from build123d import *

# Parameters (mm, degrees)
EXTRUDE_1_DEPTH     = 100
SKETCH_2_R          = 11.5
EXTRUDE_2_DEPTH     = 10
SKETCH_3_W          = 23
SKETCH_3_H          = 11.5
EXTRUDE_3_DEPTH     = 20
FILLET_3_R          = 4
FILLET_4_R          = 4
CUT_EXTRUDE_1_DEPTH = 132.291660154
EXTRUDE_4_DEPTH     = 11.5
CUT_EXTRUDE_2_DEPTH = 20
CUT_EXTRUDE_3_DEPTH = 5
SKETCH_8_R          = 1.5
CUT_EXTRUDE_4_DEPTH = 133.303102986


with BuildPart() as part:
    # 草图1 → 凸台-拉伸1 (new body)
    with BuildSketch(Plane.XY):
        with BuildLine():
            Line((-7.5, 12.990381057), (7.5, 12.990381057))
            ThreePointArc((7.5, 12.990381057), (10.606601718, 10.606601718), (12.990381057, 7.5))
            Line((12.990381057, 7.5), (12.990381057, -7.5))
            ThreePointArc((12.990381057, -7.5), (10.606601718, -10.606601718), (7.5, -12.990381057))
            Line((7.5, -12.990381057), (-7.5, -12.990381057))
            ThreePointArc((-7.5, -12.990381057), (-10.606601718, -10.606601718), (-12.990381057, -7.5))
            Line((-12.990381057, -7.5), (-12.990381057, 7.5))
            ThreePointArc((-12.990381057, 7.5), (-10.606601718, 10.606601718), (-7.5, 12.990381057))
        make_face()
    extrude(amount=EXTRUDE_1_DEPTH)

    # 草图2 → 凸台-拉伸2 (add)
    with BuildSketch(Plane.XY.offset(100)):
        Circle(SKETCH_2_R)
    extrude(amount=EXTRUDE_2_DEPTH)

    # 草图3 → 凸台-拉伸3 (add)
    with BuildSketch(Plane.XY.offset(110)):
        with Locations((0, -5.75)):
            Rectangle(SKETCH_3_W, SKETCH_3_H)
    extrude(amount=EXTRUDE_3_DEPTH)

    # 圆角3
    # the kernel refuses this fillet: 4 mm, written as the material it adds along each edge
    with BuildSketch(Plane(origin=(0, 0, 110), x_dir=(0, -1, 0), z_dir=(-1, 0, 0))) as fillet_3_piece_1_section:
        with BuildLine():
            CenterArc((11.5 + FILLET_3_R, -FILLET_3_R), FILLET_3_R, 90, 90)
            Line((11.5 + FILLET_3_R, 0), (11.5, 0))
            Line((11.5, 0), (11.5, -FILLET_3_R))
        make_face()
    fillet_3_piece_1 = revolve(axis=Axis((0, 0, 110), (0, 0, 1)), revolution_arc=90, mode=Mode.PRIVATE)
    fillet_3_piece_1 = split(fillet_3_piece_1, bisect_by=Plane(origin=(8.245599316, -11.5, 108.963397676), z_dir=(0, 1, 0)), keep=Keep.TOP, mode=Mode.PRIVATE)
    fillet_3_piece_1 = split(fillet_3_piece_1, bisect_by=Plane(origin=(11.5, -8.245600634, 108.963397676), z_dir=(-1, 0, 0)), keep=Keep.TOP, mode=Mode.PRIVATE)
    add(fillet_3_piece_1)

    # 圆角4
    # the kernel refuses this fillet: 4 mm, written as the material it adds along each edge
    with BuildSketch(Plane(origin=(0, 0, 110), x_dir=(-1, 0, 0), z_dir=(0, 1, 0))) as fillet_4_piece_1_section:
        with BuildLine():
            CenterArc((11.5 + FILLET_4_R, -FILLET_4_R), FILLET_4_R, 90, 90)
            Line((11.5 + FILLET_4_R, 0), (11.5, 0))
            Line((11.5, 0), (11.5, -FILLET_4_R))
        make_face()
    fillet_4_piece_1 = revolve(axis=Axis((0, 0, 110), (0, 0, 1)), revolution_arc=139.842431039, mode=Mode.PRIVATE)
    fillet_4_piece_1 = split(fillet_4_piece_1, bisect_by=Plane(origin=(-8.245600113, -11.5, 108.963397741), z_dir=(0, 1, 0)), keep=Keep.TOP, mode=Mode.PRIVATE)
    fillet_4_piece_1 = split(fillet_4_piece_1, bisect_by=Plane(origin=(11.5, -8.245601202, 108.963397741), z_dir=(-1, 0, 0)), keep=Keep.TOP, mode=Mode.PRIVATE)
    fillet_4_piece_1 = split(fillet_4_piece_1, bisect_by=Plane(origin=(-11.5, -8.245601202, 108.963397741), z_dir=(1, 0, 0)), keep=Keep.TOP, mode=Mode.PRIVATE)
    add(fillet_4_piece_1)

    # 草图4 → 切除-拉伸1 (cut, through all)
    with BuildSketch(Plane(origin=(0, 0, 0), x_dir=(1, 0, 0), z_dir=(0, 1, 0))):
        Polygon((3.705771366, -130), (11.5, -125.5), (11.5, -130), align=None)
        Polygon((-11.5, -130), (-3.705771366, -130), (-11.5, -125.5), align=None)
    extrude(amount=-CUT_EXTRUDE_1_DEPTH, mode=Mode.SUBTRACT)

    # 草图5 → 凸台-拉伸4 (add)
    with BuildSketch(Plane(origin=(0, 0, 0), x_dir=(1, 0, 0), z_dir=(0, 1, 0))):
        Polygon((11.5, -125.5), (16.746857011, -122.470725692), (11.5, -119.441451384), align=None)
    extrude(amount=-EXTRUDE_4_DEPTH)

    # 草图6 → 切除-拉伸2 (cut)
    with BuildSketch(Plane(origin=(0, 0, 0), x_dir=(1, 0, 0), z_dir=(0, 1, 0))):
        with BuildLine():
            Line((11.5, -114.720725692), (11.5, -119.441451384))
            ThreePointArc((11.5, -119.441451384), (10.137243875, -117.081088538), (11.5, -114.720725692))
        make_face()
    extrude(amount=-CUT_EXTRUDE_2_DEPTH, mode=Mode.SUBTRACT)

    # 草图7 → 切除-拉伸3 (cut)
    with BuildSketch(Plane(origin=(0, 0, 0), x_dir=(1, 0, 0), z_dir=(0, 1, 0))):
        with BuildLine():
            Line((16.746857011, -122.470725692), (8.086602973, -127.470725692))
            Line((8.086602973, -127.470725692), (1.102060707, -123.438198334))
            ThreePointArc((1.102060707, -123.438198334), (-2.508596349, -122.470725692), (1.102060707, -121.50325305))
            Line((1.102060707, -121.50325305), (8.086602973, -117.470725692))
            Line((8.086602973, -117.470725692), (16.746857011, -122.470725692))
        make_face()
    extrude(amount=-CUT_EXTRUDE_3_DEPTH, mode=Mode.SUBTRACT)

    # 草图8 → 切除-拉伸4 (cut, through all)
    with BuildSketch(Plane(origin=(0, -5, 0), x_dir=(1, 0, 0), z_dir=(0, 1, 0))):
        with Locations(Location((9.926348936, -122.470725692, 0), (0, 0, 270))):
            Circle(SKETCH_8_R)
    extrude(amount=-CUT_EXTRUDE_4_DEPTH, mode=Mode.SUBTRACT)


solid = part.part
Can you work these out from the model? Positions are in its coordinate system, mm. A direction names the side the tool comes from. Give positions to 0.01 mm unless a question says otherwise; leave off trailing zeros. Loops run counter-clockwise (first coordinate to the right, second up) from the corner with the lowest first, then second, coordinate; pieces in that order, holes last. Notation, with made-up numbers: (2.25, -29) -> (28.25, -29) arc R17 cw to (28.25, -15) -> close; hole circle Ø3 at (84, -37). An arc over 180 degrees is marked (long way). Return JSON: item names as keys, results as strings.
Q1. I want a section at A-A, the plane z = 60.5. List the corners of the cut face in (x, y) for me, then the cut area to 3 significant figures.
Checks:
{"outline": "(-12.99, -7.5) arc R15 ccw to (-7.5, -12.99) -> (7.5, -12.99) arc R15 ccw to (12.99, -7.5) -> (12.99, 7.5) arc R15 ccw to (7.5, 12.99) -> (-7.5, 12.99) arc R15 ccw to (-12.99, 7.5) -> close", "area": "625 mm2"}
Q2. We'd pull the mould along X, two halves only. Please class faces 1 (the face through (4.545, -2.465, 119.515)), 2 (the face through (-10.645, 10.568, 49.3)), 3 (the face through (-3, 0, 118)): released by +X, released by -X, zero draft, split by the parting line, or undercut.
Checks:
{"face 1": "undercut", "face 2": "released by -X", "face 3": "zero draft"}
Q3. I need wall thicknesses on probe 1 along Z at (x, y) = (10, -10); probe 2 along X at (y, z) = (-6.5, 12); probe 3 along Z at (x, y) = (9.25, 5.5). Which ranges of each line are inside material? Lowest first, please.
Checks:
{"probe 1": "z = 0 to 100, 109.76 to 120.97, 123.97 to 126.37", "probe 2": "x = -12.99 to 12.99", "probe 3": "z = 0 to 110"}
Q4. I want a section at B-B, the plane y = 5.5. List the corners of the cut face in (x, z) for me.
Checks:
{"outline": "(-12.99, 0) -> (12.99, 0) -> (12.99, 100) -> (10.1, 100) -> (10.1, 110) -> (-10.1, 110) -> (-10.1, 100) -> (-12.99, 100) -> close"}
Q5. On a 3-axis mill with a long thin cutter (end or side, diameter ignored), from which of +Z, -Z, +X, -X, +Y, -Y can I reach the whole of each face in a straight line? I mean faces 4 (the face through (14.2, -8.2, 121)), 5 (the face through (7, -5, 122)), 6 (the face through (-10.568, -10.645, 49.3)). Say none if no direction works.
Checks:
{"face 4": "+X, +Y, -Y", "face 5": "+Y", "face 6": "-Z, -X, -Y"}
Q6. For pin 1 Ø9 at (y, z) = (-8, 111) entering from -X; pin 2 Ø3 at (x, y) = (-3, 5) entering from +Z; pin 3 Ø4 at (x, y) = (1, 1) entering from +Z; pin 4 Ø12 at (x, z) = (7.5, 112) entering from -Y, each with a flat end and sliding along its axis, tell me the tip position at first contact or that it passes through.
Checks:
{"pin 1": "stops at x = -11.5", "pin 2": "stops at z = 110", "pin 3": "stops at z = 130", "pin 4": "stops at y = -11.5"}
